Verification items for the finished model (mm, model axes). Face numbers are marked on the shaded views. A direction names the side the tool comes from. Round coordinates to 2 decimals unless told otherwise and drop trailing zeros. Order: outer loops, then holes, each group sorted by start corner. A loop starts at its lowest first (then second) coordinate and runs counter-clockwise, first axis right, second up. Notation, with made-up numbers: (66.25, 27.5) -> (101.25, 27.5) arc R18 ccw to (101.25, 40.5) -> close; hole circle Ø3 at (9, 53). An arc over 180 degrees is marked (long way). Return JSON: item names as keys, results as strings. Group by question number.
1) Scan lines: L1, parallel to Y at x = 44.5, z = 10; L2, parallel to Y at x = 37, z = 2; L3, parallel to Y at x = 31, z = 11. Record each from-to range of solid material in increasing order.
2) Section check B-B on z = 8.25. Enter the section's corners in (x, y), plus the area to 3 significant figures.
3) Depth check by flat-ended pin: pin 1 (8 mm diameter, centred on y = 106.5, z = 7, fed in from +X); pin 2 (2 mm diameter, centred on x = 29.5, z = 6.5, fed in from +Y); pin 3 (1.7 mm diameter, centred on y = 123, z = 7.5, fed in from -X); pin 4 (6.5 mm diameter, centred on x = 44.5, z = 6, fed in from -Y). Enter the tip coordinate at first touch or a pass-through.
4) Tool access check on the marked faces 1 and 2. Record the directions out of +Z, -Z, +X, -X, +Y, -Y that give a thin tool (end or side, any length) a straight path to the whole face; none if there is none.
5) Section check C-C on y = 110. Enter the section's corners in (x, z), plus the area to 3 significant figures.
6) Section check A-A on x = 41.5. State how many separate pieces and enclosed holes the cut face has, plus the area to 3 significant figures.
7) Section check D-D on x = 33.5. Enter the section's corners in (y, z), plus the area to 3 significant figures.
```python
from build123d import *

# Parameters (mm, degrees)
BOSS_EXTRU_1_DEPTH      = 1.6
ESQUISSE3_R             = 1.148870596
ESQUISSE3_R_2           = 1.140783705
ESQUISSE3_R_3           = 1.172524647
ESQUISSE3_R_4           = 1.134797555
ENL_V_MAT_EXTRU_1_DEPTH = 1.6
COMPOSANTS_W            = 12.858194584
COMPOSANTS_H            = 12.858194584
COMPOSANTS_W_2          = 12.824969275
COMPOSANTS_H_2          = 7.30956798
COMPOSANTS_W_3          = 3.854135844
COMPOSANTS_H_3          = 4.252839552
BOSS_EXTRU_2_DEPTH      = 0.5
USB_W                   = 19.229644045
USB_H                   = 5.768893213
USB_W_2                 = 20.923684115
USB_H_2                 = 15.017436302
BOSS_EXTRU_3_DEPTH      = 13.55
ESQUISSE6_W             = 5.080672097
ESQUISSE6_H             = 10.850248885
ENL_V_MAT_EXTRU_2_DEPTH = 13.55
ESQUISSE7_W             = 3.121599382
ESQUISSE7_H             = 4.951502468
ENL_V_MAT_EXTRU_3_DEPTH = 13.55
ESQUISSE8_W             = 12.034303823
ESQUISSE8_H             = 4.628578393
ENL_V_MAT_EXTRU_4_DEPTH = 13.55
ESQUISSE9_W             = 11.539153577
ESQUISSE9_H             = 1.442394197
BOSS_EXTRU_4_DEPTH      = 13.55
CONG_1_R                = 0.25


with BuildPart() as part:
    # plaque → Boss.-Extru.1 (new body)
    with BuildSketch(Plane.XY):
        with BuildLine():
            Line((43.900262464, 135.755357431), (5.620539516, 135.755357431))
            ThreePointArc((5.620539516, 135.755357431), (3.852772563, 135.023124384), (3.120539516, 133.255357431))
            Line((3.120539516, 133.255357431), (3.120539516, 95.39098691))
            ThreePointArc((3.120539516, 95.39098691), (3.852772563, 93.623219957), (5.620539516, 92.89098691))
            Line((5.620539516, 92.89098691), (43.900262464, 92.89098691))
            ThreePointArc((43.900262464, 92.89098691), (45.668029417, 93.623219957), (46.400262464, 95.39098691))
            Line((46.400262464, 95.39098691), (46.400262464, 133.255357431))
            ThreePointArc((46.400262464, 133.255357431), (45.668029417, 135.023124384), (43.900262464, 135.755357431))
        make_face()
    extrude(amount=-BOSS_EXTRU_1_DEPTH)

    # Esquisse3 → Enlèv. mat.-Extru.1 (cut)
    with BuildSketch(Plane.XY):
        with Locations((5.759516269, 133.070860948)):
            Circle(ESQUISSE3_R)
        with Locations((5.683227949, 95.539332189)):
            Circle(ESQUISSE3_R_2)
        with Locations((43.653009493, 132.961233721)):
            Circle(ESQUISSE3_R_3)
        with Locations((43.659821284, 95.506212136)):
            Circle(ESQUISSE3_R_4)
    extrude(amount=-ENL_V_MAT_EXTRU_1_DEPTH, mode=Mode.SUBTRACT)

    # composants → Boss.-Extru.2 (add)
    with BuildSketch(Plane.XY):
        with Locations((21.530912713, 117.16211726)):
            Rectangle(COMPOSANTS_W, COMPOSANTS_H)
        with Locations((15.832772219, 103.822155695)):
            Rectangle(COMPOSANTS_W_2, COMPOSANTS_H_2)
        with Locations((10.749299941, 127.079871998)):
            Rectangle(COMPOSANTS_W_3, COMPOSANTS_H_3)
    extrude(amount=BOSS_EXTRU_2_DEPTH)

    # usb → Boss.-Extru.3 (add)
    with BuildSketch(Plane.XY):
        with Locations((39.921367739, 123.990139203)):
            Rectangle(USB_W, USB_H)
        with Locations((39.074347704, 110.071539704)):
            Rectangle(USB_W_2, USB_H_2)
    extrude(amount=BOSS_EXTRU_3_DEPTH)

    # Esquisse6 → Enlèv. mat.-Extru.2 (cut)
    with BuildSketch(Plane(origin=(49.536189761, 0, 0), x_dir=(0, 0, -1), z_dir=(1, 0, 0))):
        with Locations((-8.79520358, 110.082102666)):
            Rectangle(ESQUISSE6_W, ESQUISSE6_H)
    extrude(amount=-ENL_V_MAT_EXTRU_2_DEPTH, mode=Mode.SUBTRACT)

    # Esquisse7 → Enlèv. mat.-Extru.3 (cut)
    with BuildSketch(Plane(origin=(49.536189761, 0, 0), x_dir=(0, 0, -1), z_dir=(1, 0, 0))):
        with Locations((-4.69406784, 110.060574394)):
            Rectangle(ESQUISSE7_W, ESQUISSE7_H)
    extrude(amount=-ENL_V_MAT_EXTRU_3_DEPTH, mode=Mode.SUBTRACT)

    # Esquisse8 → Enlèv. mat.-Extru.4 (cut)
    with BuildSketch(Plane(origin=(49.536189761, 0, 0), x_dir=(0, 0, -1), z_dir=(1, 0, 0))):
        with Locations((-6.933008087, 123.957073711)):
            Rectangle(ESQUISSE8_W, ESQUISSE8_H)
    extrude(amount=-ENL_V_MAT_EXTRU_4_DEPTH, mode=Mode.SUBTRACT)

    # Esquisse9 → Boss.-Extru.4 (add)
    with BuildSketch(Plane(origin=(35.986189761, 0, 0), x_dir=(0, 0, -1), z_dir=(1, 0, 0))):
        with Locations((-6.922243951, 122.579264329)):
            Rectangle(ESQUISSE9_W, ESQUISSE9_H)
    extrude(amount=BOSS_EXTRU_4_DEPTH)

    # Congé1
    cong_1_edges = [part.edges().sort_by_distance(p)[0] for p in [
        (39.921367738, 121.105692596, 13.55),
        (39.921367738, 126.874585809, 13.55),
    ]]
    fillet(cong_1_edges, radius=CONG_1_R)


solid = part.part
```
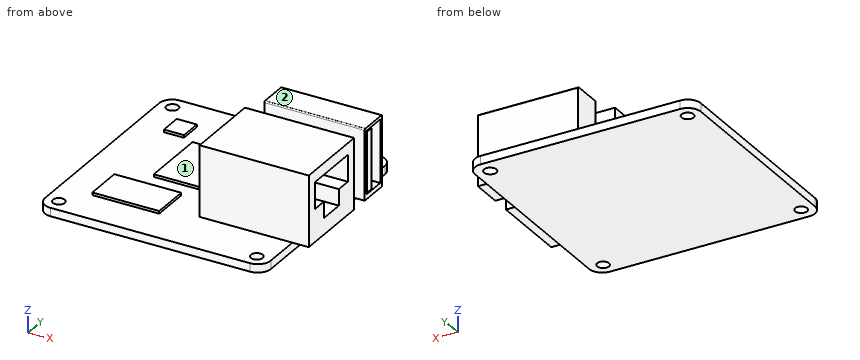
Check result:
{
 "1": {"L1": "102.56 to 104.66, 115.51 to 117.58, 121.11 to 121.64, 121.86 to 123.3, 126.27 to 126.87", "L2": "102.56 to 117.58, 121.11 to 121.64, 121.86 to 123.3, 126.27 to 126.87", "L3": "102.56 to 117.58, 121.11 to 126.87"},
 "2": {"outline": "(28.61, 102.56) -> (49.54, 102.56) -> (49.54, 104.66) -> (35.99, 104.66) -> (35.99, 115.51) -> (49.54, 115.51) -> (49.54, 117.58) -> (28.61, 117.58) -> close; (30.31, 121.11) -> (49.54, 121.11) -> (49.54, 121.64) -> (35.99, 121.64) -> (35.99, 121.86) -> (49.54, 121.86) -> (49.54, 123.3) -> (35.99, 123.3) -> (35.99, 126.27) -> (49.54, 126.27) -> (49.54, 126.87) -> (30.31, 126.87) -> close", "area": "235 mm^2"},
 "3": {"pin 1": "x = 49.54", "pin 2": "y = 126.87", "pin 3": "x = 30.31", "pin 4": "y = 102.56"},
 "4": {"face 1": "+Z, -X, +Y, -Y", "face 2": "+Z, +X, -X, +Y, -Y"},
 "5": {"outline": "(3.12, -1.6) -> (46.4, -1.6) -> (46.4, 0) -> (49.54, 0) -> (49.54, 3.13) -> (35.99, 3.13) -> (35.99, 11.34) -> (49.54, 11.34) -> (49.54, 13.55) -> (28.61, 13.55) -> (28.61, 0) -> (3.12, 0) -> close", "area": "242 mm^2"},
 "6": {"separate pieces": "2", "enclosed holes": "2", "area": "241 mm^2"},
 "7": {"outline": "(92.89, -1.6) -> (135.76, -1.6) -> (135.76, 0) -> (126.87, 0) -> (126.87, 13.3) arc R0.25 ccw to (126.62, 13.55) -> (121.36, 13.55) arc R0.25 ccw to (121.11, 13.3) -> (121.11, 0) -> (117.58, 0) -> (117.58, 13.55) -> (102.56, 13.55) -> (102.56, 0) -> (92.89, 0) -> close", "area": "350 mm^2"}
}
